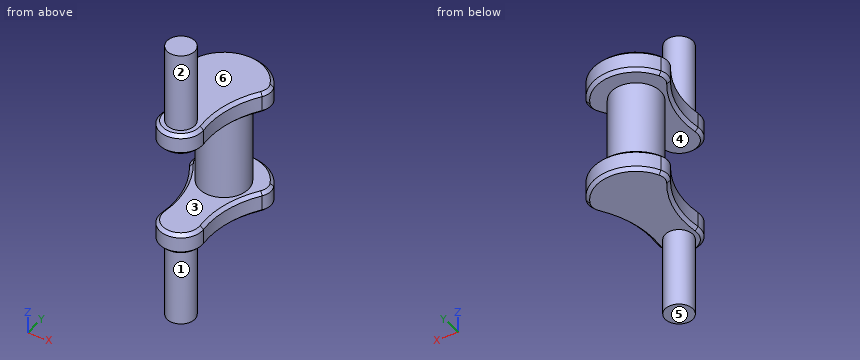
from build123d import *

# Parameters (mm, degrees)
SKETCH1_R                = 23
BOSS_EXTRUDE1_DEPTH      = 40
BOSS_EXTRUDE2_DEPTH      = 20
SKETCH3_R                = 13
BOSS_EXTRUDE3_DEPTH      = 75
FILLET1_R                = 15
CHAMFER2_SIZE            = 3
FILLET1_OF_MIRROR1_R     = 15
CHAMFER2_OF_MIRROR1_SIZE = 3


with BuildPart() as part:
    # Sketch1 → Boss-Extrude1 (new body, symmetric)
    with BuildSketch(Plane.XY):
        Circle(SKETCH1_R)
    extrude(amount=BOSS_EXTRUDE1_DEPTH, both=True)

    # Sketch2 → Boss-Extrude2 (add)
    with BuildSketch(Plane.XY.offset(40)):
        with BuildLine():
            ThreePointArc((39.051840285, 8.657584558), (0, 40), (-39.051840285, 8.657584558))
            ThreePointArc((-39.051840285, 8.657584558), (-22.47215166, -23.418781152), (-19.834213041, -59.430176458))
            ThreePointArc((-19.834213041, -59.430176458), (0, -82), (19.834213041, -59.430176458))
            ThreePointArc((19.834213041, -59.430176458), (22.47215166, -23.418781152), (39.051840285, 8.657584558))
        make_face()
    boss_extrude2 = extrude(amount=BOSS_EXTRUDE2_DEPTH)

    # Sketch3 → Boss-Extrude3 (add)
    with BuildSketch(Plane.XY.offset(60)):
        with Locations(Location((0, -62, 0), (0, 0, 180))):  # turned: the seam where the file's is
            Circle(SKETCH3_R)
    boss_extrude3 = extrude(amount=BOSS_EXTRUDE3_DEPTH)

    # Fillet1
    fillet1_edges = [part.edges().sort_by_distance(p)[0] for p in [
        (-39.051840285, 8.657584558, 50),
        (39.051840285, 8.657584558, 50),
    ]]
    fillet(fillet1_edges, radius=FILLET1_R)

    # Chamfer2
    chamfer2_edges = [part.edges().sort_by_distance(p)[0] for p in [
        (-21.554755506, -26.939885243, 40),
        (-21.554755506, -26.939885243, 60),
        (0, 40, 40),
        (37.287308792, 10.281927657, 40),
        (-37.287308792, 10.281927657, 40),
        (0, 40, 60),
        (37.287308792, 10.281927657, 60),
        (-37.287308792, 10.281927657, 60),
        (0, -82, 40),
        (21.554755506, -26.939885243, 40),
        (0, -82, 60),
        (21.554755506, -26.939885243, 60),
    ]]
    chamfer(chamfer2_edges, length=CHAMFER2_SIZE)

    # Mirror1: Boss-Extrude2, Boss-Extrude3 across plane
    add(boss_extrude2.mirror(Plane.XY))
    add(boss_extrude3.mirror(Plane.XY))

    # Fillet1 of Mirror1
    fillet1_of_mirror1_edges = [part.edges().sort_by_distance(p)[0] for p in [
        (-39.051840285, 8.657584558, -50),
        (39.051840285, 8.657584558, -50),
    ]]
    fillet(fillet1_of_mirror1_edges, radius=FILLET1_OF_MIRROR1_R)

    # Chamfer2 of Mirror1
    chamfer2_of_mirror1_edges = [part.edges().sort_by_distance(p)[0] for p in [
        (-21.554755506, -26.939885243, -40),
        (-21.554755506, -26.939885243, -60),
        (0, 40, -40),
        (37.287308792, 10.281927657, -40),
        (-37.287308792, 10.281927657, -40),
        (0, 40, -60),
        (37.287308792, 10.281927657, -60),
        (-37.287308792, 10.281927657, -60),
        (0, -82, -40),
        (21.554755506, -26.939885243, -40),
        (0, -82, -60),
        (21.554755506, -26.939885243, -60),
    ]]
    chamfer(chamfer2_of_mirror1_edges, length=CHAMFER2_OF_MIRROR1_SIZE)


solid = part.part
Source: CAD feature listing. Evaluate the final solid. Frame: model axes, mm. Face numbers are marked on the shaded views. A direction names the side the tool comes from. Give positions to 0.01 mm unless a question says otherwise; leave off trailing zeros. Write each loop counter-clockwise with the first axis right and the second up, starting at its lowest first coordinate (ties: lowest second). Pieces come first, ordered by that corner, then holes. Notation, with made-up numbers: (38.5, 88.25) -> (67.5, 88.25) arc R27 cw to (67.5, 123.25) -> close; hole circle Ø10 at (21.25, -19). An arc over 180 degrees is marked (long way). Return JSON: item names as keys, results as strings. Group by question number.
1. Material intervals for line 1 (Z direction, x = 24, y = 26); line 2 (Z direction, x = -10.5, y = 3); line 3 (Z direction, x = -17, y = -45), sorted ascending. Write a range as from..to.
2. Section C-C, the plane z = 10.5. Output: boundary loops of the cut face in (x, y).
3. Mould query, pull axis Z, two halves, no side actions, for the marked faces 4, 5 and 6. Classes: +Z half, -Z half, draft (parallel to the pull), parting line (faces both ways), or undercut.
4. Access query for the marked faces 1, 2 and 3. Directions: +Z, -Z, +X, -X, +Y, -Y. A direction counts if a zero-diameter tool reaches every point of the face in a straight line with its end or side. Return the directions, or none.
5. Section A-A, the plane x = 0. Output: boundary loops of the cut face in (y, z), then the cut area to 3 significant figures.
6. Pin query (flat end, axial travel): pin 1 Ø20.5 at (x, y) = (-9.5, -19.5) entering from +Z; pin 2 Ø10 at (y, z) = (11, -48) entering from -X; pin 3 Ø10 at (y, z) = (-42, 34.5) entering from +X; pin 4 Ø2 at (x, y) = (-29, 20) entering from -Z. Return the tip coordinate at first contact, or that it passes through.
7. Section B-B, the plane z = 103.5. Output: boundary loops of the cut face in (x, y).
Determined:
{
 "1": {"line 1": "z = -60..-40, 40..60", "line 2": "z = -60..60", "line 3": "z = -59.13..-40.87, 40.87..59.13"},
 "2": {"outline": "circle Ø46 at (0, 0)"},
 "3": {"face 4": "undercut", "face 5": "-Z half", "face 6": "+Z half"},
 "4": {"face 1": "-Z", "face 2": "+Z", "face 3": "none"},
 "5": {"outline": "(-82, -57) -> (-79, -60) -> (-75, -60) -> (-75, -135) -> (-49, -135) -> (-49, -60) -> (37, -60) -> (40, -57) -> (40, -43) -> (37, -40) -> (23, -40) -> (23, 40) -> (37, 40) -> (40, 43) -> (40, 57) -> (37, 60) -> (-49, 60) -> (-49, 135) -> (-75, 135) -> (-75, 60) -> (-79, 60) -> (-82, 57) -> (-82, 43) -> (-79, 40) -> (-23, 40) -> (-23, -40) -> (-79, -40) -> (-82, -43) -> close", "area": "12,400 mm2"},
 "6": {"pin 1": "stops at z = 60", "pin 2": "stops at x = -37.32", "pin 3": "passes through", "pin 4": "stops at z = -60"},
 "7": {"outline": "circle Ø26 at (0, -62)"}
}
